Can you work these out from the model? Positions are in its coordinate system, mm. Face numbers are marked on the shaded views. Coordinates: 2 decimals unless noted, no trailing zeros. Write each loop counter-clockwise with the first axis right and the second up, starting at its lowest first coordinate (ties: lowest second). Pieces come first, ordered by that corner, then holes. Notation, with made-up numbers: (-37, 23) -> (1, 23) arc R18 cw to (1, 58) -> close; hole circle Ø9 at (79.25, 44.25). An arc over 180 degrees is marked (long way). Use one line per item in the form item = value.
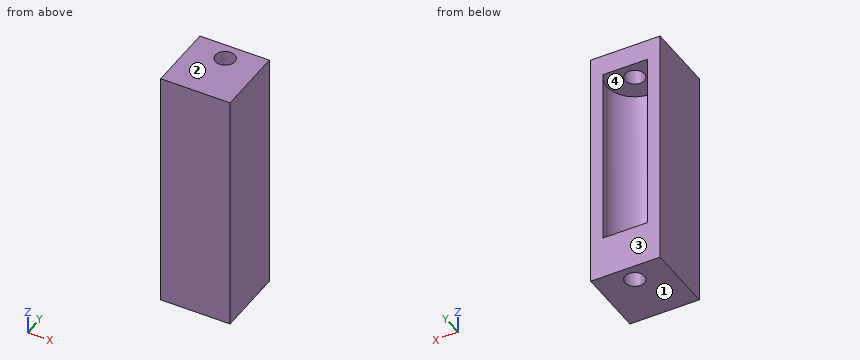
```python
from build123d import *

# Parameters (mm, degrees)
F0_W     = 50
F0_H     = 176
F1_DEPTH = 50
F2_R     = 7
F3_DEPTH = 176.001
F4_START = -15
F4_DEPTH = 130


with BuildPart() as f1:
    # F0 (on Front) → F1 (new body)
    with BuildSketch(Plane.XZ):
        with Locations((25, 88)):
            Rectangle(F0_W, F0_H)
    extrude(amount=-F1_DEPTH)

    # F2 (on face) → F3 (cut, through all)
    with BuildSketch(Plane.XY.offset(176)):
        with Locations((25, 38)):
            Circle(F2_R)
    extrude(amount=-F3_DEPTH, mode=Mode.SUBTRACT)

    # F2 (on face) → F4 (cut)
    with BuildSketch(Plane.XY.offset(176).offset(F4_START)):
        with BuildLine():
            ThreePointArc((9, 50), (18.6754446797, 19.026334039), (45, 38))
            ThreePointArc((45, 38), (43.973665961, 44.3245553203), (41, 50))
            Line((41, 50), (9, 50))
        make_face()
        with Locations((25, 38)):
            Circle(F2_R, mode=Mode.SUBTRACT)
    extrude(amount=-F4_DEPTH, mode=Mode.SUBTRACT)


solid = f1.part
```
Q1. Suppose I cut it at B-B (y = 34). Write out the boundary of the cut face in (x, z), then the cut area to 3 significant figures.
Return value:
outline = (0, 0) -> (19.26, 0) -> (19.26, 31) -> (5.4, 31) -> (5.4, 161) -> (19.26, 161) -> (19.26, 176) -> (0, 176) -> close; (30.74, 0) -> (50, 0) -> (50, 176) -> (30.74, 176) -> (30.74, 161) -> (44.6, 161) -> (44.6, 31) -> (30.74, 31) -> close
area = 3,180 mm2
Q2. Thinking about a two-plate mould opening in Z: for the marked faces 1, 2, 3 and 4, which applies, released by +Z, released by -Z, zero draft, split by the parting line, or undercut?
Return value:
face_1 = released by -Z
face_2 = released by +Z
face_3 = zero draft
face_4 = undercut
Q3. Suppose I cut it at D-D (z = 21). Write out the boundary of the cut face in (x, y).
Return value:
outline = (0, 0) -> (50, 0) -> (50, 50) -> (0, 50) -> close; hole circle Ø14 at (25, 38)
Q4. Suppose I cut it at C-C (z = 93). Write out the boundary of the cut face in (x, y), then the cut area to 3 significant figures.
Return value:
outline = (0, 0) -> (50, 0) -> (50, 50) -> (41, 50) arc R20 cw (long way) to (9, 50) -> (0, 50) -> close
area = 1,420 mm2
Q5. Will these pins go through, and if not, where does the flat tip stop? pin 1 (4 mm diameter, centred on x = 17.5, z = 158, fed in from +Y); pin 2 (10 mm diameter, centred on x = 15, z = 151.5, fed in from +Y).
Return value:
pin_1 = 20.4
pin_2 = 24.77
Q6. Suppose I cut it at A-A (x = 25). Write out the boundary of the cut face in (y, z), then the cut area to 3 significant figures.
Return value:
outline = (0, 0) -> (31, 0) -> (31, 31) -> (18, 31) -> (18, 161) -> (31, 161) -> (31, 176) -> (0, 176) -> close; (45, 0) -> (50, 0) -> (50, 31) -> (45, 31) -> close; (45, 161) -> (50, 161) -> (50, 176) -> (45, 176) -> close
area = 4,000 mm2
Q7. If I drill on line 1 (Y direction, x = 25, z = 171); line 2 (X direction, y = 38, z = 108); line 3 (Z direction, x = 21, y = 26), over which ranges is the centre line in solid material (lowest first)? Write a range as from..to.
Return value:
line_1 = 0..31, 45..50
line_2 = 0..5, 45..50
line_3 = 0..31, 161..176
